Input: part model. Units: mm. Frame: model coordinates. A direction names the side the tool comes from. Coordinates: 2 decimals unless noted, no trailing zeros. Loops run counter-clockwise (first coordinate to the right, second up) from the corner with the lowest first, then second, coordinate; pieces in that order, holes last. Notation, with made-up numbers: (56, 24) -> (69, 24) arc R14 ccw to (69, 49) -> close; hole circle Ø4 at (-16, -10). An arc over 180 degrees is marked (long way). Put each result on its own line as item: value. Start each with the question number.
1) Cut plane B-B (z = -100). Return the cut outline in (x, y), plus the area to 3 significant figures.
2) Pull-direction query (Z, two-part tool) for faces 3 (the flat face through (-5, 10, -4)), 4 (the flat face through (-354.72, 5.07, 186.385)); classes: pulls with the +Z half, pulls with the -Z half, needs draft (parallel to the pull), parting line crosses it, or undercut.
3) Contact query for a flat-ended pin moving along its axis: P1, Ø4, axis at y = 8.5, z = -166, coming from the -X side. Output: stop coordinate, or through.
4) Material intervals for L1, parallel to Z at x = -305, y = 7.75; L2, parallel to X at y = 7.5, z = -125; L3, parallel to X at y = 6.75, z = -37.5, sorted ascending.
5) Cut plane A-A (y = 4.5). Return the cut outline in (x, z), plus the area to 3 significant figures.
6) Set-up query: faces 1 (the flat face through (-355.28, 5.07, -186.71)), 2 (the flat face through (-5, 0, -4)). Return all of +Z, -Z, +X, -X, +Y, -Y with unobstructed straight access to the full face (end or side cutting, diameter ignored); none if empty.
from build123d import *

# Parameters (mm, degrees)
SKETCH1_W           = 750
SKETCH1_H           = 500
BOSS_EXTRUDE1_DEPTH = 10
SKETCH2_R           = 4
CUT_EXTRUDE1_DEPTH  = 10
SKETCH3_R           = 4
CUT_EXTRUDE2_DEPTH  = 10
SKETCH4_R           = 4
CUT_EXTRUDE3_DEPTH  = 10
SKETCH5_R           = 4
CUT_EXTRUDE4_DEPTH  = 10
SKETCH6_R           = 4
CUT_EXTRUDE5_DEPTH  = 10
SKETCH7_R           = 4
CUT_EXTRUDE6_DEPTH  = 10
CUT_EXTRUDE7_REACH  = 12


with BuildPart() as part:
    # Sketch1 → Boss-Extrude1 (new body)
    with BuildSketch(Plane(origin=(0, 0, 0), x_dir=(1, 0, 0), z_dir=(0, 1, 0))):
        Rectangle(SKETCH1_W, SKETCH1_H)
    extrude(amount=BOSS_EXTRUDE1_DEPTH)

    # Sketch2 → Cut-Extrude1 (cut)
    with BuildSketch(Plane(origin=(0, 10, 0), x_dir=(1, 0, 0), z_dir=(0, 1, 0))):
        with Locations((305, 125)):
            Circle(SKETCH2_R)
    extrude(amount=-CUT_EXTRUDE1_DEPTH, mode=Mode.SUBTRACT)

    # Sketch3 → Cut-Extrude2 (cut)
    with BuildSketch(Plane(origin=(0, 10, 0), x_dir=(1, 0, 0), z_dir=(0, 1, 0))):
        with Locations((305, -125)):
            Circle(SKETCH3_R)
    extrude(amount=-CUT_EXTRUDE2_DEPTH, mode=Mode.SUBTRACT)

    # Sketch4 → Cut-Extrude3 (cut)
    with BuildSketch(Plane(origin=(0, 10, 0), x_dir=(1, 0, 0), z_dir=(0, 1, 0))):
        with Locations((0, 125)):
            Circle(SKETCH4_R)
    extrude(amount=-CUT_EXTRUDE3_DEPTH, mode=Mode.SUBTRACT)

    # Sketch5 → Cut-Extrude4 (cut)
    with BuildSketch(Plane(origin=(0, 10, 0), x_dir=(1, 0, 0), z_dir=(0, 1, 0))):
        with Locations((0, -125)):
            Circle(SKETCH5_R)
    extrude(amount=-CUT_EXTRUDE4_DEPTH, mode=Mode.SUBTRACT)

    # Sketch6 → Cut-Extrude5 (cut)
    with BuildSketch(Plane(origin=(0, 10, 0), x_dir=(1, 0, 0), z_dir=(0, 1, 0))):
        with Locations((-305, 125)):
            Circle(SKETCH6_R)
    extrude(amount=-CUT_EXTRUDE5_DEPTH, mode=Mode.SUBTRACT)

    # Sketch7 → Cut-Extrude6 (cut)
    with BuildSketch(Plane(origin=(0, 10, 0), x_dir=(1, 0, 0), z_dir=(0, 1, 0))):
        with Locations((-305, -125)):
            Circle(SKETCH7_R)
    extrude(amount=-CUT_EXTRUDE6_DEPTH, mode=Mode.SUBTRACT)

    # Sketch10 → Cut-Extrude7 (cut, up to next)
    with BuildSketch(Plane(origin=(0, 10, 0), x_dir=(1, 0, 0), z_dir=(0, 1, 0)), mode=Mode.PRIVATE) as cut_extrude7_sk1:
        Polygon((-335, 175), (-335, -175), (-375, -198.094010768), (-375, 198.094010768), align=None)
    cut_extrude7_tool1 = extrude(cut_extrude7_sk1.sketch, amount=-CUT_EXTRUDE7_REACH, mode=Mode.PRIVATE) & part.part
    add(cut_extrude7_tool1.solids().sort_by_distance((-355.412658, 10, 0))[0], mode=Mode.SUBTRACT)


solid = part.part
Results found:
1. outline: (-335, 0) -> (375, 0) -> (375, 10) -> (-335, 10) -> close
1. area: 7,100 mm2
2. face 3: needs draft
2. face 4: undercut
3. P1: stops at x = -335
4. L1: z = -250 to -129, -121 to 121, 129 to 250
4. L2: x = -335 to -309, -301 to -4, 4 to 301, 309 to 375
4. L3: x = -335 to 375
5. outline: (-375, -250) -> (375, -250) -> (375, 250) -> (-375, 250) -> (-375, 198.09) -> (-335, 175) -> (-335, -175) -> (-375, -198.09) -> close; hole circle Ø8 at (-305, -125); hole circle Ø8 at (-305, 125); hole circle Ø8 at (0, -125); hole circle Ø8 at (0, 125); hole circle Ø8 at (305, -125); hole circle Ø8 at (305, 125)
5. area: 360,000 mm2
6. face 1: -X, +Y, -Y
6. face 2: +Z, -Z, +X, -X, -Y
